Can you work these out from the drawing? Everything is in mm from the part's minimum corner. A direction names the side the tool comes from. Round coordinates to 2 decimals unless told otherwise and drop trailing zeros. Write each loop counter-clockwise with the first axis right and the second up, starting at its lowest first coordinate (ties: lowest second). Pieces come first, ordered by that corner, then holes. Notation, with made-up numbers: (-17.75, 58.25) - (-8.75, 58.25) arc R13 ccw to (-8.75, 81.25) - close; hole circle Ø5 at (82, 44). An arc over 180 degrees is marked (long way). One line per item, written item: value. Start each with the question number.
Item 1: If I drill on line 1 (Z direction, x = 13, y = 7); line 2 (Y direction, x = 5, z = 5.25); line 3 (X direction, y = 7.5, z = 13), over which ranges is the centre line in solid material (lowest first)?
Item 2: Thinking about a two-plate mould opening in Z: for the marked faces 6, 7, 8 and 9, which applies, released by +Z, released by -Z, zero draft, split by the parting line, or undercut?
Item 3: For P1, Ø5, axis at y = 7.5, z = 21, coming from the -X side; P2, Ø3.5, axis at x = 55, y = 5, coming from the +Z side; P3, Ø1.5, axis at x = 34.5, y = 5, coming from the +Z side, each with a flat end and sliding along its axis, tell me the tip position at first contact or that it passes through.
Item 4: For the marked faces 1, 2, 3, 4 and 5, which set-ups out of +Z, -Z, +X, -X, +Y, -Y let a thin tool reach every point of the face, with its end or its side?
Item 5: Imagine slicing it at C-C, the plane z = 24.5. Please give me the cut outline in (x, y), then the cut area to 3 significant figures.
Item 6: Imagine slicing it at D-D, the plane x = 34.5. Please give me the cut outline in (y, z), then the cut area to 3 significant figures.
Item 7: Imagine slicing it at B-B, the plane x = 5. Please give me the cut outline in (y, z), then the cut area to 3 significant figures.
Item 8: Imagine slicing it at A-A, the plane x = 52. Please give me the cut outline in (y, z), then the cut area to 3 significant figures.
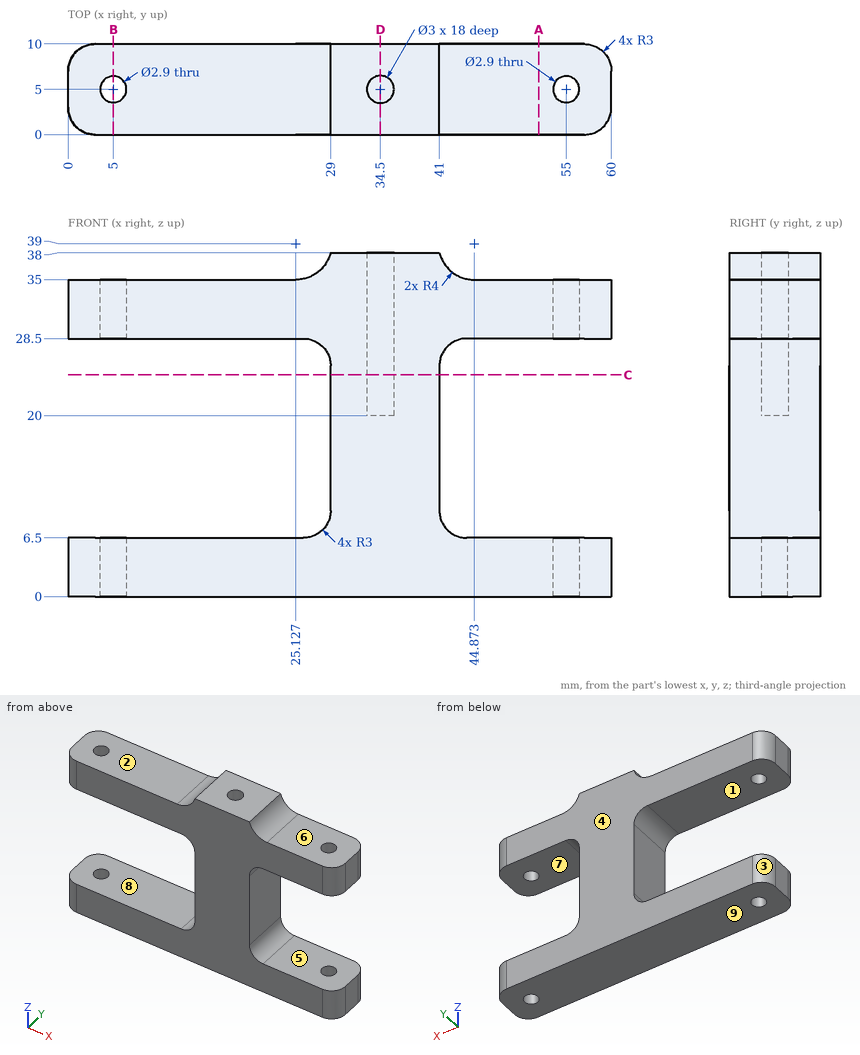
Values follow:
1. line 1: z = 0 to 6.5, 28.5 to 35
1. line 2: y = 0 to 3.55, 6.45 to 10
1. line 3: x = 29 to 41
2. face 6: released by +Z
2. face 7: undercut
2. face 8: undercut
2. face 9: released by -Z
3. P1: stops at x = 29
3. P2: stops at z = 35
3. P3: stops at z = 20
4. face 1: -X, +Y, -Y
4. face 2: +Z, -X, +Y, -Y
4. face 3: +Z, -Z, -X, +Y
4. face 4: +Z, -Z, +X, -X, +Y
4. face 5: +X, +Y, -Y
5. outline: (29, 0) - (41, 0) - (41, 10) - (29, 10) - close; hole circle Ø3 at (34.5, 5)
5. area: 113 mm^2
6. outline: (0, 0) - (10, 0) - (10, 38) - (6.5, 38) - (6.5, 20) - (3.5, 20) - (3.5, 38) - (0, 38) - close
6. area: 326 mm^2
7. outline: (0, 0) - (3.55, 0) - (3.55, 6.5) - (0, 6.5) - close; (0, 28.5) - (3.55, 28.5) - (3.55, 35) - (0, 35) - close; (6.45, 0) - (10, 0) - (10, 6.5) - (6.45, 6.5) - close; (6.45, 28.5) - (10, 28.5) - (10, 35) - (6.45, 35) - close
7. area: 92.3 mm^2
8. outline: (0, 0) - (10, 0) - (10, 6.5) - (0, 6.5) - close; (0, 28.5) - (10, 28.5) - (10, 35) - (0, 35) - close
8. area: 130 mm^2
